Source: CAD feature listing. Evaluate the final solid. Frame: model axes, mm. Face numbers are marked on the shaded views. A direction names the side the tool comes from. Give positions to 0.01 mm unless a question says otherwise; leave off trailing zeros. Order: outer loops, then holes, each group sorted by start corner. A loop starts at its lowest first (then second) coordinate and runs counter-clockwise, first axis right, second up.
1) First-contact query: P1, Ø6.5, axis at y = 2.5, z = 11, coming from the -X side; P2, Ø4, axis at x = 22, z = 13, coming from the +Y side; P3, Ø6.5, axis at y = 9, z = 5, coming from the +X side. Flat tips, straight axial feed; report the tip coordinate or a pass-through.
2) Section A-A, the plane x = 22. Return loops of the section in (y, z), plus the area to 3 significant figures.
3) Material intervals for line 1 (X direction, y = 2.35, z = 13); line 2 (Y direction, x = 2.5, z = 14.75); line 3 (X direction, y = 6.5, z = 9.25), sorted ascending.
4) Section C-C, the plane z = 6.75. Return loops of the section in (x, y), plus the area to 3 significant figures.
5) Section B-B, the plane z = 13. Return loops of the section in (x, y).
6) Access query for the marked faces 1, 2, 3 and 4. Directions: +Z, -Z, +X, -X, +Y, -Y. A direction counts if a zero-diameter tool reaches every point of the face in a straight line with its end or side. Return the directions, or none.
7) Section D-D, the plane y = 5.5. Return loops of the section in (x, z), plus the area to 3 significant figures.
```python
from build123d import *

# Parameters (mm, degrees)
BOSS_EXTRUDE1_DEPTH = 10
SKETCH3_W           = 26
SKETCH3_H           = 4
BOSS_EXTRUDE2_DEPTH = 17
SKETCH4_R           = 1.5
CUT_EXTRUDE1_DEPTH  = 4


with BuildPart() as part:
    # Sketch1 → Boss-Extrude1 (new body)
    with BuildSketch(Plane.XY):
        with BuildLine():
            Line((0.947795447, 55.867567374), (-5.354013975, 64.102890964))
            ThreePointArc((-5.354013975, 64.102890964), (-14.235235054, 34.948420067), (0, 8))
            Line((0, 8), (0, 4))
            Line((0, 4), (12, 4))
            Line((12, 4), (12, 12))
            ThreePointArc((12, 12), (-3.507060252, 31.419133439), (0.947795447, 55.867567374))
        make_face()
    extrude(amount=BOSS_EXTRUDE1_DEPTH)

    # Sketch3 → Boss-Extrude2 (add)
    with BuildSketch(Plane.XY):
        with Locations((13, 2)):
            Rectangle(SKETCH3_W, SKETCH3_H)
    extrude(amount=BOSS_EXTRUDE2_DEPTH)

    # Sketch4 → Cut-Extrude1 (cut)
    with BuildSketch(Plane(origin=(0, 4, 0), x_dir=(1, 0, 0), z_dir=(0, 1, 0))):
        with Locations(Location((4, -13, 0), (0, 0, 270))):
            Circle(SKETCH4_R)
        with Locations(Location((10, -13, 0), (0, 0, 270))):
            Circle(SKETCH4_R)
        with Locations(Location((16, -13, 0), (0, 0, 270))):
            Circle(SKETCH4_R)
        with Locations(Location((22, -13, 0), (0, 0, 270))):
            Circle(SKETCH4_R)
    extrude(amount=-CUT_EXTRUDE1_DEPTH, mode=Mode.SUBTRACT)


solid = part.part
```
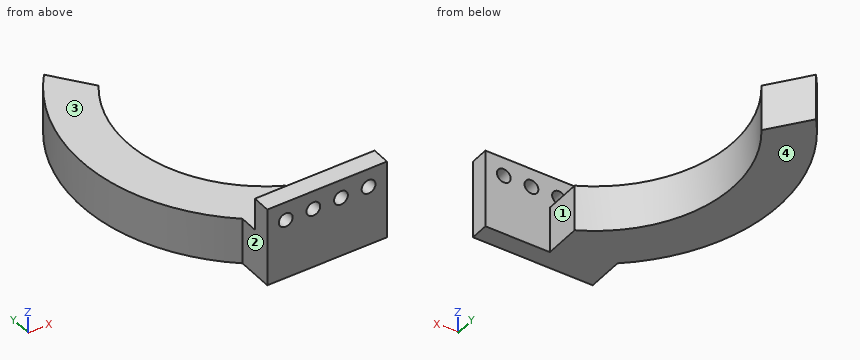
From the geometry:
1. P1: stops at x = 0
1. P2: stops at y = 4
1. P3: stops at x = 12
2. outline: (0, 0) - (4, 0) - (4, 11.5) - (0, 11.5) - close; (0, 14.5) - (4, 14.5) - (4, 17) - (0, 17) - close
2. area: 56.0 mm2
3. line 1: x = 0 to 2.5, 5.5 to 8.5, 11.5 to 14.5, 17.5 to 20.5, 23.5 to 26
3. line 2: y = 0 to 4
3. line 3: x = 0 to 12
4. outline: (-5.35, 64.1) arc R40 ccw to (0, 8) - (0, 0) - (26, 0) - (26, 4) - (12, 4) - (12, 12) arc R30 cw to (0.95, 55.87) - close
4. area: 744 mm2
5. outline: (0, 0) - (2.5, 0) - (2.5, 4) - (0, 4) - close; (5.5, 0) - (8.5, 0) - (8.5, 4) - (5.5, 4) - close; (11.5, 0) - (14.5, 0) - (14.5, 4) - (11.5, 4) - close; (17.5, 0) - (20.5, 0) - (20.5, 4) - (17.5, 4) - close; (23.5, 0) - (26, 0) - (26, 4) - (23.5, 4) - close
6. face 1: +Z, -Z, +X, +Y
6. face 2: +Z, -Z, -X, -Y
6. face 3: +Z, +X, -X, +Y
6. face 4: -Z, +X, -X, +Y, -Y
7. outline: (0, 0) - (12, 0) - (12, 10) - (0, 10) - close
7. area: 120 mm2
